```python
from build123d import *

# Parameters (mm, degrees)
SKETCH1_W           = 16
SKETCH1_H           = 21
SKETCH1_R           = 1.8
BOSS_EXTRUDE2_DEPTH = 5
SKETCH2_R           = 2.66
CUT_EXTRUDE1_DEPTH  = 3


with BuildPart() as part:
    # Sketch1 → Boss-Extrude2 (new body)
    with BuildSketch(Plane(origin=(0, 0, 0), x_dir=(1, 0, 0), z_dir=(0, 1, 0))):
        Rectangle(SKETCH1_W, SKETCH1_H)
        with Locations(Location((0, 5.2, 0), (0, 0, 270))):
            Circle(SKETCH1_R, mode=Mode.SUBTRACT)
    extrude(amount=BOSS_EXTRUDE2_DEPTH)

    # Sketch2 → Cut-Extrude1 (cut)
    with BuildSketch(Plane(origin=(0, 5, 0), x_dir=(1, 0, 0), z_dir=(0, 1, 0))):
        with Locations((-8, 5.2)):
            Circle(SKETCH2_R)
        with Locations((8, 5.2)):
            Circle(SKETCH2_R)
    extrude(amount=-CUT_EXTRUDE1_DEPTH, mode=Mode.SUBTRACT)


solid = part.part
```
Check sheet for the modelled part. Datum: model origin and axes. Units: mm. A direction names the side the tool comes from. Give positions to 0.01 mm unless a question says otherwise; leave off trailing zeros. Write each loop counter-clockwise with the first axis right and the second up, starting at its lowest first coordinate (ties: lowest second). Pieces come first, ordered by that corner, then holes. Notation, with made-up numbers: (83.5, 75.5) -> (106.5, 75.5) arc R22 ccw to (106.5, 108.5) -> close; hole circle Ø3 at (38, 1.5). An arc over 180 degrees is marked (long way). Use CSV: the item, a comma, the result in double quotes. Start each with the question number.
Q1. Tool access check on faces 1 (the cylindrical face through (5.34, 3.52, -5.26)), 2 (the cylindrical face through (0.541, 2.465, -3.483)), 3 (the cylindrical face through (-5.34, 3.52, -5.14)). Record the directions out of +Z, -Z, +X, -X, +Y, -Y that give a thin tool (end or side, any length) a straight path to the whole face; none if there is none.
Q2. Cross-section at A-A on z = -5.2. Enter the section's corners in (x, y).
Q3. Depth check by flat-ended pin: P1, Ø1, axis at y = 2.5, z = -3, coming from the +X side; P2, Ø2, axis at x = -7, z = -6, coming from the +Y side. Enter the tip coordinate at first touch or a pass-through.
Q4. Cross-section at C-C on x = -7. Enter the section's corners in (y, z), and give its area (3 significant figures).
Q5. Cross-section at B-B on y = 3.5. Enter the section's corners in (x, z), and give its area (3 significant figures).
Q6. Cross-section at D-D on y = 1.2. Enter the section's corners in (x, z).
Q7. Scan lines: line 1 along X through (y, z) = (2.2, -5.2); line 2 along Z through (x, y) = (-1.5, 1.3); line 3 along Z through (x, y) = (6.75, 4.65). Record each from-to range of solid material in increasing order.
Working result:
1,face 1,"+X, +Y"
1,face 2,"+Y, -Y"
1,face 3,"-X, +Y"
2,outline,"(-8, 0) -> (-1.8, 0) -> (-1.8, 5) -> (-5.34, 5) -> (-5.34, 2) -> (-8, 2) -> close; (1.8, 0) -> (8, 0) -> (8, 2) -> (5.34, 2) -> (5.34, 5) -> (1.8, 5) -> close"
3,P1,"stops at x = 8"
3,P2,"stops at y = 2"
4,outline,"(0, -10.5) -> (5, -10.5) -> (5, -7.66) -> (2, -7.66) -> (2, -2.74) -> (5, -2.74) -> (5, 10.5) -> (0, 10.5) -> close"
4,area,"90.2 mm^2"
5,outline,"(-8, -10.5) -> (8, -10.5) -> (8, -7.86) arc R2.66 cw to (8, -2.54) -> (8, 10.5) -> (-8, 10.5) -> (-8, -2.54) arc R2.66 cw to (-8, -7.86) -> close; hole circle Ø3.6 at (0, -5.2)"
5,area,"304 mm^2"
6,outline,"(-8, -10.5) -> (8, -10.5) -> (8, 10.5) -> (-8, 10.5) -> close; hole circle Ø3.6 at (0, -5.2)"
7,line 1,"x = -5.34 to -1.8, 1.8 to 5.34"
7,line 2,"z = -10.5 to -6.19, -4.21 to 10.5"
7,line 3,"z = -10.5 to -7.55, -2.85 to 10.5"
